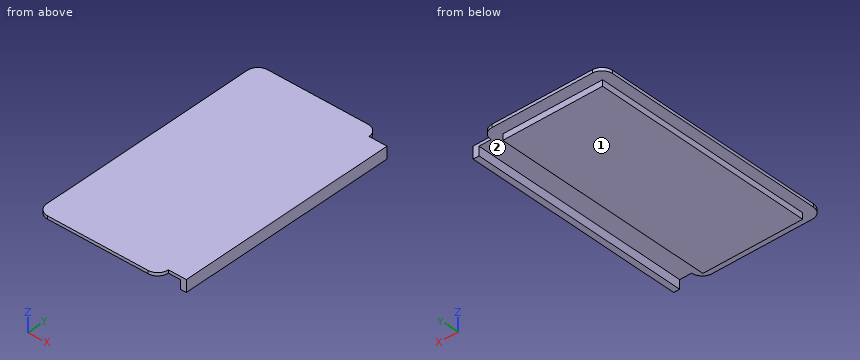
Autodesk Fusion 360 part; units mm, degrees
sketch "Sketch1" plane through (0, 0, 0) normal (0, 0, 1) x (1, 0, 0)
  line L0 (-50.8, 101.6) -> (50.8, 101.6)
  line L1 (50.8, 101.6) -> (50.8, -101.6)
  line L2 (50.8, -101.6) -> (-50.8, -101.6)
  line L3 (-50.8, -101.6) -> (-50.8, 101.6)
  line L4 (-50.8, 101.6) -> (50.8, -101.6) construction
  line L5 (50.8, 101.6) -> (-50.8, -101.6) construction
  dimension "d1" = 101.6
  dimension "d2" = 203.2
extrude "Extrude1" add sketch "Sketch1" along normal blind 2.54
fillet "Fillet1" radius 8.89 4 edges at (-50.8, -101.6, 1.27) (50.8, -101.6, 1.27) (50.8, 101.6, 1.27) (-50.8, 101.6, 1.27)
extrude "Extrude4" add 1 faces at (50.8, 30.9033, 0.8467) along direction (1, 0, 0) blind 10
sketch "Sketch3" plane through (0, 0, 2.54) normal (0, 0, 1) x (-1, 0, 0)
  arc A0 (41.91, -101.6) -> (50.8, -92.71) centre (41.91, -92.71) ccw
  line L0 (50.8, -92.71) -> (50.8, 92.71)
  arc A1 (50.8, 92.71) -> (41.91, 101.6) centre (41.91, 92.71) ccw
  line L1 (41.91, 101.6) -> (-41.91, 101.6)
  arc A2 (-41.91, 101.6) -> (-50.8, 92.71) centre (-41.91, 92.71) ccw
  line L2 (-50.8, 92.71) -> (-60.8, 92.71)
  line L3 (-60.8, 92.71) -> (-60.8, -92.71)
  line L4 (-60.8, -92.71) -> (-50.8, -92.71)
  arc A3 (-50.8, -92.71) -> (-41.91, -101.6) centre (-41.91, -92.71) ccw
  line L5 (-41.91, -101.6) -> (41.91, -101.6)
  line L6 (-60.8, -92.71) -> (-65.8, -92.71)
  line L7 (-65.8, -92.71) -> (-65.8, 92.71)
  line L8 (-65.8, 92.71) -> (-60.8, 92.71)
  line L9 (-60.8, 92.71) -> (-60.8, -92.71)
  dimension "d28" = 5
extrude "Extrude5" add sketch "Sketch3" against normal blind 10 contours L3 L6 L7 L8 L9
sketch "Sketch4" plane through (0, 0, 0) normal (0, 0, -1) x (1, 0, 0)
  arc A0 (-50.8, -92.71) -> (-41.91, -101.6) centre (-41.91, -92.71) ccw
  line L0 (-41.91, -101.6) -> (41.91, -101.6)
  arc A1 (41.91, -101.6) -> (50.8, -92.71) centre (41.91, -92.71) ccw
  line L1 (50.8, -92.71) -> (60.8, -92.71)
  line L2 (60.8, -92.71) -> (60.8, 92.71)
  line L3 (60.8, 92.71) -> (50.8, 92.71)
  arc A2 (50.8, 92.71) -> (41.91, 101.6) centre (41.91, 92.71) ccw
  line L4 (41.91, 101.6) -> (-41.91, 101.6)
  arc A3 (-41.91, 101.6) -> (-50.8, 92.71) centre (-41.91, 92.71) ccw
  line L5 (-50.8, 92.71) -> (-50.8, -92.71)
  line L6 (50.8, -92.71) -> (50.8, 92.71) construction
  line L7 (-41.91, 92.71) -> (41.4111, 92.71)
  line L8 (41.4111, 92.71) -> (41.4111, -92.21)
  line L9 (41.4111, -92.21) -> (-41.91, -92.21)
  line L10 (-41.91, -92.21) -> (-41.91, 92.71)
  line L11 (-41.91, 92.71) -> (41.4111, -92.21) construction
  line L12 (41.4111, 92.71) -> (-41.91, -92.21) construction
  point P0 (-0.2495, 0.25)
  dimension "d32" = 184.92
  dimension "d36" = 83.3211
extrude "Extrude6" add sketch "Sketch4" along normal blind 5 contours L7 L8 L9 L10
equation "d32 = 185.42 mm - 0.5 mm"
equation "d36 = 83.82109398 mm - 0.5 mm"
Read the model definition and answer for the solid it produces. Units are mm, in the model's axes. Face numbers are marked on the shaded views. Give positions to 0.01 mm unless a question says otherwise; leave off trailing zeros. Write each loop counter-clockwise with the first axis right and the second up, starting at its lowest first coordinate (ties: lowest second). Pieces come first, ordered by that corner, then holes. Notation, with made-up numbers: (-18, 13) -> (0, 13) arc R17 ccw to (0, 36) -> close; hole circle Ø5 at (-32.75, 11.25). An arc over 180 degrees is marked (long way). Answer in a Markdown table with one row per item.
1) Section B-B on y = 68.5 is taken. Give the vertices of the cut face in (x, z), plus the area to 3 significant figures.
Results list:
| item | result |
|---|---|
| outline | (-50.8, 0) -> (-41.91, 0) -> (-41.91, -5) -> (41.41, -5) -> (41.41, 0) -> (60.8, 0) -> (60.8, -7.46) -> (65.8, -7.46) -> (65.8, 2.54) -> (-50.8, 2.54) -> close |
| area | 750 mm^2 |
2) Each of these flat-tipped pins is pushed along its axis until it touches: pin 1 Ø1.5 at (x, z) = (-2, -2.5) entering from -Y; pin 2 Ø2.5 at (x, z) = (7, -3) entering from +Y; pin 3 Ø1 at (x, y) = (-2, 79) entering from -Z. Where does it stop, or does it pass through?
Results list:
| item | result |
|---|---|
| pin 1 | y = -92.71 |
| pin 2 | y = 92.21 |
| pin 3 | z = -5 |
3) Section A-A on z = -2.75 is taken. Give the vertices of the cut face in (x, y), plus the area to 3 significant figures.
Results list:
| item | result |
|---|---|
| outline | (-41.91, -92.71) -> (41.41, -92.71) -> (41.41, 92.21) -> (-41.91, 92.21) -> close; (60.8, -92.71) -> (65.8, -92.71) -> (65.8, 92.71) -> (60.8, 92.71) -> close |
| area | 16,300 mm^2 |
4) Determine the mould class of the marked faces 1 and 2 for opening direction X: released by +X, released by -X, zero draft, split by the parting line, or undercut.
Results list:
| item | result |
|---|---|
| face 1 | zero draft |
| face 2 | undercut |
5) Straight lines are drawn through the part: line 1 (X direction, y = 63.5, z = -3.75); line 2 (Y direction, x = -7.5, z = -0.75); line 3 (X direction, y = -5, z = -6). For each, find the intervals that lie inside material, in ascending order. Write a range as [from, to].
Results list:
| item | result |
|---|---|
| line 1 | [-41.91, 41.41], [60.8, 65.8] |
| line 2 | [-92.71, 92.21] |
| line 3 | [60.8, 65.8] |
6) Section D-D on x = 56.5 is taken. Give the vertices of the cut face in (y, z).
Results list:
| item | result |
|---|---|
| outline | (-92.71, 0) -> (92.71, 0) -> (92.71, 2.54) -> (-92.71, 2.54) -> close |
7) Section C-C on x = 20.5 is taken. Give the vertices of the cut face in (y, z).
Results list:
| item | result |
|---|---|
| outline | (-101.6, 0) -> (-92.71, 0) -> (-92.71, -5) -> (92.21, -5) -> (92.21, 0) -> (101.6, 0) -> (101.6, 2.54) -> (-101.6, 2.54) -> close |
